Input: dimensioned drawing with shaded views. Units: mm. Origin: part minimum x, y, z. Give positions to 0.01 mm unless a question says otherwise; leave off trailing zeros. Loops run counter-clockwise (first coordinate to the right, second up) from the corner with the lowest first, then second, coordinate; pieces in that order, holes last. Notation, with made-up numbers: (-39, 56.25) -> (-31, 56.25) arc R14 ccw to (-31, 66.25) -> close; hole circle Ø2 at (9, 6.25). An arc over 180 degrees is marked (long way). Answer in a Markdown table with one row per item. Add a question column.
1) Section query C-C (y = 3). Give the number of separate pieces and of enclosed holes in the cut face, plus the area to 3 significant figures.
2) Section query B-B (z = 31.59). Return the cut outline in (x, y), plus the area to 3 significant figures.
3) First-contact query: P1, Ø2.5, axis at x = 40.14, z = 23.04, coming from the +Y side; P2, Ø1.5, axis at x = 47, y = 1, coming from the -Z side; P3, Ø3.5, axis at x = 40.14, z = 40.14, coming from the -Y side; P4, Ø3, axis at y = 7.5, z = 40, coming from the +X side (3 decimals). Flat tips, straight axial feed; report the tip coordinate or a pass-through.
4) Section query D-D (x = 54). Return the cut outline in (y, z).
5) Section query A-A (x = 31.59). Return the cut outline in (y, z).
6) Line query: line 1 (Z direction, x = 31.59, y = 2.5); line 2 (Z direction, x = 23.04, y = 7.25); line 3 (Z direction, x = 22.5, y = 4.25). Output: solid intervals per line, ascending. Write a range as from..to.
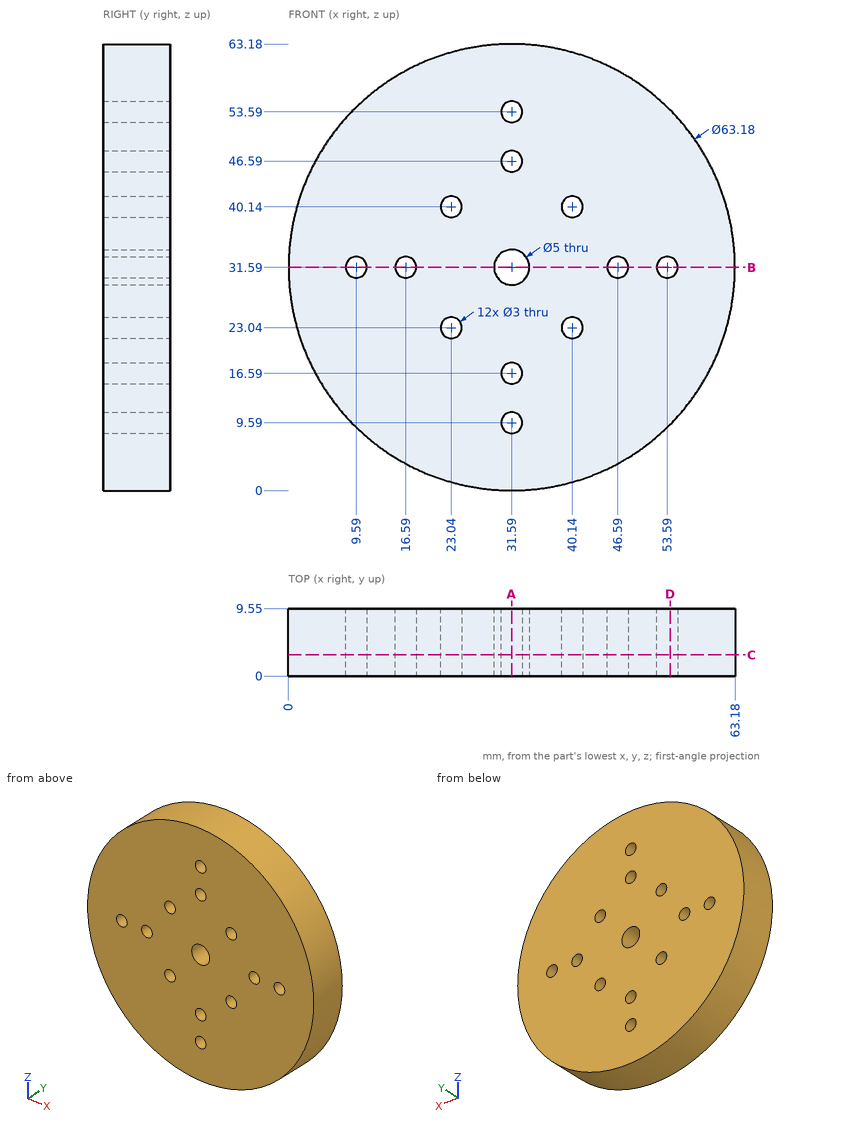
Evaluation:
| question | item | result |
|---|---|---|
| 1 | separate pieces | 1 |
| 1 | enclosed holes | 13 |
| 1 | area | 3,030 mm² |
| 2 | outline | (0, 0) -> (8.09, 0) -> (8.09, 9.55) -> (0, 9.55) -> close; (11.09, 0) -> (15.09, 0) -> (15.09, 9.55) -> (11.09, 9.55) -> close; (18.09, 0) -> (29.09, 0) -> (29.09, 9.55) -> (18.09, 9.55) -> close; (34.09, 0) -> (45.09, 0) -> (45.09, 9.55) -> (34.09, 9.55) -> close; (48.09, 0) -> (52.09, 0) -> (52.09, 9.55) -> (48.09, 9.55) -> close; (55.09, 0) -> (63.18, 0) -> (63.18, 9.55) -> (55.09, 9.55) -> close |
| 2 | area | 441 mm² |
| 3 | P1 | through |
| 3 | P2 | z = 3.61 |
| 3 | P3 | y = 0 |
| 3 | P4 | x = 62.415 |
| 4 | outline | (0, 9.33) -> (9.55, 9.33) -> (9.55, 30.15) -> (0, 30.15) -> close; (0, 33.03) -> (9.55, 33.03) -> (9.55, 53.85) -> (0, 53.85) -> close |
| 5 | outline | (0, 0) -> (9.55, 0) -> (9.55, 8.09) -> (0, 8.09) -> close; (0, 11.09) -> (9.55, 11.09) -> (9.55, 15.09) -> (0, 15.09) -> close; (0, 18.09) -> (9.55, 18.09) -> (9.55, 29.09) -> (0, 29.09) -> close; (0, 34.09) -> (9.55, 34.09) -> (9.55, 45.09) -> (0, 45.09) -> close; (0, 48.09) -> (9.55, 48.09) -> (9.55, 52.09) -> (0, 52.09) -> close; (0, 55.09) -> (9.55, 55.09) -> (9.55, 63.18) -> (0, 63.18) -> close |
| 6 | line 1 | 0..8.09, 11.09..15.09, 18.09..29.09, 34.09..45.09, 48.09..52.09, 55.09..63.18 |
| 6 | line 2 | 1.18..21.54, 24.54..38.64, 41.64..62 |
| 6 | line 3 | 1.34..21.64, 24.44..38.74, 41.54..61.84 |
